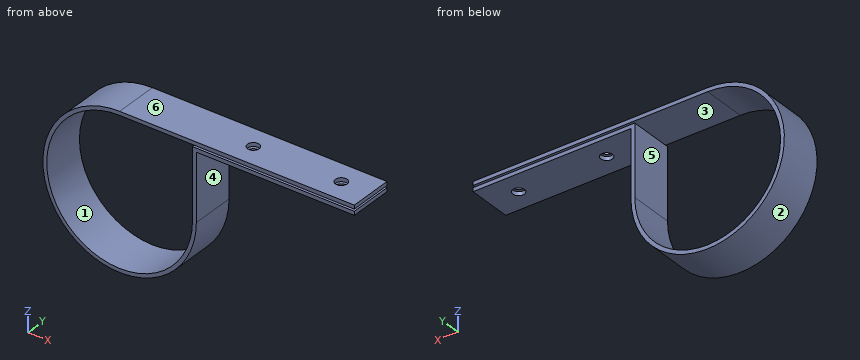
from build123d import *

# Parameters (mm, degrees)
SKETCH2_W          = 1.651
SKETCH2_H          = 19.05
SKETCH3_R          = 2.54
CUT_EXTRUDE1_DEPTH = 5.191001743


with BuildPart() as part:
    # Sweep1: sweep along a path in Sketch1
    with BuildLine(Plane(origin=(0, 0, 0), x_dir=(1, 0, 0), z_dir=(0, 1, 0))) as sweep1_path:
        Line((0, 0), (-101.6, 0))
        ThreePointArc((-101.6, 0), (-124.514215323, 55.280847216), (-69.225758741, 32.384998213))
        Line((-69.225758741, 32.384998213), (-69.225758741, 2.54))
        Line((-69.225758741, 2.54), (0, 2.54))
    # Sketch2 → Sweep1 (sweep)
    with BuildSketch(Plane(origin=(0, 0, 0), x_dir=(0, 0, -1), z_dir=(1, 0, 0))):
        Rectangle(SKETCH2_W, SKETCH2_H)
    sweep(path=sweep1_path.line, transition=Transition.RIGHT)

    # Sketch3 → Cut-Extrude1 (cut, through all)
    with BuildSketch(Plane(origin=(0, 0, -3.3655), x_dir=(-1, 0, 0), z_dir=(0, 0, -1))):
        with Locations((50.787439211, 0)):
            Circle(SKETCH3_R)
        with Locations((12.687439211, 0)):
            Circle(SKETCH3_R)
    extrude(amount=-CUT_EXTRUDE1_DEPTH, mode=Mode.SUBTRACT)


solid = part.part
Could you check a few things on this model? Use its own coordinates, in mm. Face numbers are marked on the shaded views. A direction names the side the tool comes from. Give positions to 0.01 mm unless a question says otherwise; leave off trailing zeros. Order: outer loops, then holes, each group sorted by start corner. A loop starts at its lowest first (then second) coordinate and runs counter-clockwise, first axis right, second up.
1. Suppose I cut it at B-B (x = -33). List the corners of the cut face in (y, z) for me (1 decimal).
2. We'd pull the mould along X, two halves only. Please class the marked faces 1, 2 and 3: pulls with the +X half, pulls with the -X half, needs draft (parallel to the pull), parting line crosses it, or undercut.
3. Suppose I cut it at A-A (y = -4.5). List the corners of the cut face in (x, z) for me (1 decimal).
4. I need wall thicknesses on L1, parallel to Z at x = -35, y = -3; L2, parallel to X at y = 7.5, z = -37; L3, parallel to X at y = -0.75, z = -25. Which ranges of each line are inside material? Lowest first, please.
5. For the marked faces 4, 5 and 6, which set-ups out of +Z, -Z, +X, -X, +Y, -Y let a thin tool reach every point of the face, with its end or its side?
6. Will these pins go through, and if not, where does the flat tip stop? P1, Ø3, axis at x = -112.5, y = -3, coming from the -Z side; P2, Ø4, axis at x = -110, y = -4.5, coming from the +Z side; P3, Ø1.5, axis at y = 7, z = -19, coming from the -X side.
7. Suppose I cut it at C-C (z = -15.5). List the corners of the cut face in (x, y) for me (3 decimals), plus the area to 3 significant figures.
Solved:
1. outline: (-9.5, -3.4) - (9.5, -3.4) - (9.5, -1.7) - (-9.5, -1.7) - close; (-9.5, -0.8) - (9.5, -0.8) - (9.5, 0.8) - (-9.5, 0.8) - close
2. face 1: undercut
2. face 2: parting line crosses it
2. face 3: needs draft
3. outline: (-101.6, -0.8) - (0, -0.8) - (0, 0.8) - (-101.6, 0.8) arc R33.2 ccw (long way) to (-68.4, -32.4) - (-68.4, -3.4) - (0, -3.4) - (0, -1.7) - (-70.1, -1.7) - (-70.1, -32.4) arc R31.6 cw (long way) to start
4. L1: z = -3.37 to -1.71, -0.83 to 0.83
4. L2: x = -134.5 to -132.83, -70.39 to -68.72
4. L3: x = -133.99 to -132.29, -70.05 to -68.4
5. face 4: -Z, +X, +Y, -Y
5. face 5: +Y, -Y
5. face 6: +Z, +X, -X, +Y, -Y
6. P1: stops at z = -64.24
6. P2: stops at z = 0.21
6. P3: stops at x = -132.32
7. outline: (-130.209, -9.525) - (-128.273, -9.525) - (-128.273, 9.525) - (-130.209, 9.525) - close; (-70.051, -9.525) - (-68.4, -9.525) - (-68.4, 9.525) - (-70.051, 9.525) - close
7. area: 68.3 mm2
